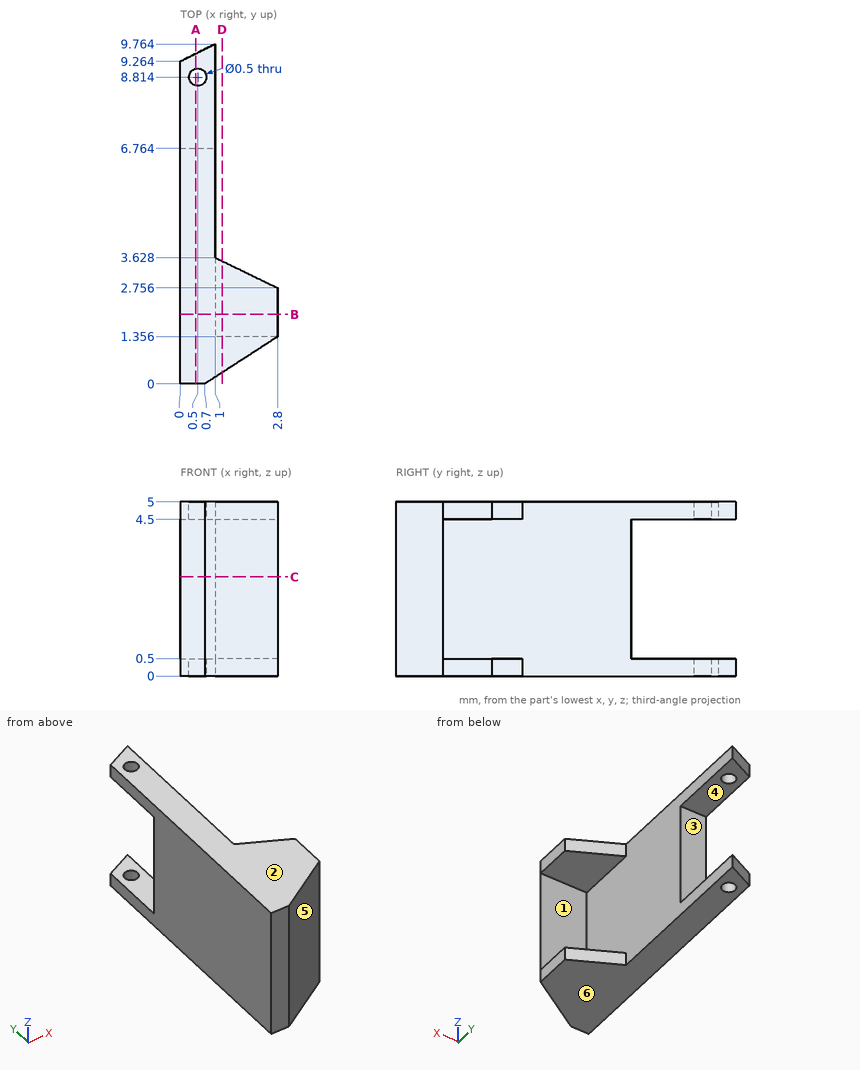
Part print with two shaded views. Sizes in mm from the minimum x, y, z corner. A direction names the side the tool comes from. Coordinates: 2 decimals unless noted, no trailing zeros. Write each loop counter-clockwise with the first axis right and the second up, starting at its lowest first coordinate (ties: lowest second). Pieces come first, ordered by that corner, then holes.
(1) Drill centre lines: line 1 (Z direction, x = 1.5, y = 2.5); line 2 (X direction, y = 3, z = 2.65); line 3 (Y direction, x = 0.5, z = 0.2) (1 decimal). Where is each one in solid material? Low to high.
(2) Mould opens along Z. For the marked faces 4, 5 and 6 say: pulls with the +Z half, pulls with the -Z half, needs draft (parallel to the pull), parting line crosses it, or undercut.
(3) Cut at A-A on x = 0.45. List the corners of the cut face in (y, z) (1 decimal).
(4) 3-axis set-ups, long thin cutter, end or side, ignore diameter. For the marked faces 1, 2 and 3: which of +Z, -Z, +X, -X, +Y, -Y reach the whole face in a straight line?
(5) Cut at C-C on z = 2.85. List the corners of the cut face in (x, y) (1 decimal).
(6) Pin check, flat tip, straight feed: pin 1 Ø0.8 at (x, z) = (0.5, 3) entering from +Y. Stop position of the tip, or through.
(7) Cut at D-D on x = 1.2. List the corners of the cut face in (y, z).
(8) Cut at B-B on y = 2. List the corners of the cut face in (x, z).
Working result:
1. line 1: z = 0 to 0.5, 4.5 to 5
1. line 2: x = 0 to 1
1. line 3: y = 0 to 8.6, 9.1 to 9.5
2. face 4: undercut
2. face 5: needs draft
2. face 6: pulls with the -Z half
3. outline: (0, 0) - (8.6, 0) - (8.6, 0.5) - (6.8, 0.5) - (6.8, 4.5) - (8.6, 4.5) - (8.6, 5) - (0, 5) - close; (9.1, 0) - (9.5, 0) - (9.5, 0.5) - (9.1, 0.5) - close; (9.1, 4.5) - (9.5, 4.5) - (9.5, 5) - (9.1, 5) - close
4. face 1: +X, +Y
4. face 2: +Z, +X, -X, +Y, -Y
4. face 3: +X, -X, +Y
5. outline: (0, 0) - (0.7, 0) - (2.8, 1.4) - (1, 1.4) - (1, 6.8) - (0, 6.8) - close
6. pin 1: stops at y = 6.76
7. outline: (0.32, 0) - (3.53, 0) - (3.53, 0.5) - (1.36, 0.5) - (1.36, 4.5) - (3.53, 4.5) - (3.53, 5) - (0.32, 5) - close
8. outline: (0, 0) - (2.8, 0) - (2.8, 0.5) - (1, 0.5) - (1, 4.5) - (2.8, 4.5) - (2.8, 5) - (0, 5) - close
